The model under review builds one solid part; all positions refer to its coordinate system, in mm. A direction names the side the tool comes from. Round coordinates to 2 decimals unless told otherwise and drop trailing zeros. Order: outer loops, then holes, each group sorted by start corner. A loop starts at its lowest first (then second) coordinate and runs counter-clockwise, first axis right, second up. Notation, with made-up numbers: M -27.5,-32.5 L 18.5,-32.5 A22 cw 18.5,-9.5 Z; hole C 47.5,89.25 d10. An arc over 180 degrees is marked long. Answer as a JSON object with one key per item and string values. Group by question number.
1) For faces 1 (the flat face through (-16, -11, 25)), 2 (the flat face through (-1, 1, 0)), list the 3-axis set-ups (+Z, -Z, +X, -X, +Y, -Y) from which the entire face can be reached by the end or side of a thin tool; tool diameter is ignored.
2) Consider section B-B, the plane y = 0. Write out the cut boundary in (x, z).
3) To check wall thickness, follow line 1 (Z direction, x = -16, y = -17); line 2 (Y direction, x = -8.5, z = 45); line 3 (X direction, y = 15, z = 43). State the ranges of each line that lie inside material, in increasing order.
4) Consider section D-D, the plane y = -21. Write out the cut boundary in (x, z), then the cut area to 3 significant figures.
5) Insertion check: pin 1 Ø5 at (x, y) = (48, 25) entering from +Z; pin 2 Ø1 at (x, z) = (13.5, 31) entering from -Y; pin 3 Ø2 at (y, z) = (-19.5, 29) entering from -X; pin 4 Ø1.5 at (x, y) = (12, 9.5) entering from -Z. Each pin has a flat end and moves straight along its axis. Give the tip position at first contact, or say it passes through.
6) Consider section A-A, the plane x = 0. Write out the cut boundary in (y, z).
7) Consider section C-C, the plane z = 41. Write out the cut boundary in (x, y), then the cut area to 3 significant figures.
```python
from build123d import *

# Parameters (mm, degrees)
F0_W     = 135.5276703835
F0_H     = 103.6717817187
F1_DEPTH = 25
F2_R     = 17.2700021185
F3_DEPTH = 25
F5_DEPTH = 103.6727817187


# Not quite as in the source:
# - a feature names something its author has since deleted; it is built from what else it names


with BuildPart() as f1:
    # F0 (on Top) → F1 (new body)
    with BuildSketch(Plane.XY):
        Rectangle(F0_W, F0_H)
    extrude(amount=F1_DEPTH)

    # F2 (on face) → F3 (join)
    with BuildSketch(Plane.XY.offset(25)):
        Circle(F2_R)
    extrude(amount=F3_DEPTH)

    # F4 (on face) → F5 (cut, through all)
    with BuildSketch(Plane.XZ.offset(51.8358908594)):
        Polygon((23.7591248006, 58.1170134246), (-17.2700021185, 50), (17.2700021185, 33.2325548289), (23.7591248006, 30.0824102014), align=None)
    extrude(amount=-F5_DEPTH, mode=Mode.SUBTRACT)


solid = f1.part
```
Results list:
{
 "1": {"face 1": "+Z", "face 2": "-Z, +X, -X, +Y, -Y"},
 "2": {"outline": "M -67.76,0 L 67.76,0 L 67.76,25 L 17.27,25 L 17.27,33.23 L -17.27,50 L -17.27,25 L -67.76,25 Z"},
 "3": {"line 1": "0 to 25", "line 2": "-15.03 to 15.03", "line 3": "-8.56 to -2.85"},
 "4": {"outline": "M -67.76,0 L 67.76,0 L 67.76,25 L -67.76,25 Z", "area": "3,390 mm^2"},
 "5": {"pin 1": "z = 25", "pin 2": "y = -11.37", "pin 3": "through", "pin 4": "z = 0"},
 "6": {"outline": "M -51.84,0 L 51.84,0 L 51.84,25 L 17.27,25 L 17.27,41.62 L -17.27,41.62 L -17.27,25 L -51.84,25 Z"},
 "7": {"outline": "M 1.27,-17.22 L 1.27,17.22 A17.27 ccw long Z", "area": "512 mm^2"}
}
